Part model, mm, in its own coordinate system. A direction names the side the tool comes from. Round coordinates to 2 decimals unless told otherwise and drop trailing zeros. Loops run counter-clockwise (first coordinate to the right, second up) from the corner with the lowest first, then second, coordinate; pieces in that order, holes last.
from build123d import *

# Parameters (mm, degrees)
SKETCH_1_R               = 30
SKETCH_1_R_2             = 2.5
EXTRUDE_1_DEPTH          = 17
SKETCH_2_R               = 16
CUT_EXTRUDE_1_DEPTH      = 18
PATTERN_CIRCULAR_1_COUNT = 3
SKETCH_4_R               = 11
EXTRUDE_3_DEPTH          = 14
SKETCH_5_R               = 5
CUT_EXTRUDE_2_DEPTH      = 32
SKETCH_6_W               = 4
SKETCH_6_H               = 2.5
CUT_EXTRUDE_3_DEPTH      = 32
SKETCH_7_R               = 13
EXTRUDE_4_DEPTH          = 4
EXTRUDE_5_DEPTH          = 35
SKETCH_10_R              = 13
SKETCH_10_R_2            = 11
EXTRUDE_8_DEPTH          = 3
FILLET_1_R               = 5


with BuildPart() as part:
    # 草图1 → 凸台-拉伸1 (new body)
    with BuildSketch(Plane.XY):
        Circle(SKETCH_1_R)
        with Locations((-5.952838037, 22.216294005)):
            Circle(SKETCH_1_R_2, mode=Mode.SUBTRACT)
        with Locations((5.952838037, 22.216294005)):
            Circle(SKETCH_1_R_2, mode=Mode.SUBTRACT)
        with Locations((22.216294005, -5.952838037)):
            Circle(SKETCH_1_R_2, mode=Mode.SUBTRACT)
        with Locations((16.263455967, -16.263455967)):
            Circle(SKETCH_1_R_2, mode=Mode.SUBTRACT)
        with Locations((-16.263455967, -16.263455967)):
            Circle(SKETCH_1_R_2, mode=Mode.SUBTRACT)
        with Locations((-22.216294005, -5.952838037)):
            Circle(SKETCH_1_R_2, mode=Mode.SUBTRACT)
    extrude(amount=EXTRUDE_1_DEPTH)

    # 草图2 → 切除-拉伸1 (cut, through all)
    with BuildSketch(Plane.XY.offset(17)):
        with Locations((25.980762114, 15)):
            Circle(SKETCH_2_R)
    cut_extrude_1 = extrude(amount=-CUT_EXTRUDE_1_DEPTH, mode=Mode.SUBTRACT)

    # 阵列(圆周)1: 切除-拉伸1 ×3 about axis
    pattern_circular_1_axis = Axis((0, 0, 0), (0, 0, 1))
    for i in range(1, PATTERN_CIRCULAR_1_COUNT):
        add(cut_extrude_1.rotate(pattern_circular_1_axis, i * 360 / PATTERN_CIRCULAR_1_COUNT), mode=Mode.SUBTRACT)

    # 草图4 → 凸台-拉伸3 (add)
    with BuildSketch(Plane.XY.offset(17)):
        Circle(SKETCH_4_R)
    extrude(amount=EXTRUDE_3_DEPTH)

    # 草图5 → 切除-拉伸2 (cut, through all)
    with BuildSketch(Plane.XY.offset(31)):
        Circle(SKETCH_5_R)
    extrude(amount=-CUT_EXTRUDE_2_DEPTH, mode=Mode.SUBTRACT)

    # 草图6 → 切除-拉伸3 (cut, through all)
    with BuildSketch(Plane.XY.offset(31)):
        with Locations((0, 5)):
            Rectangle(SKETCH_6_W, SKETCH_6_H)
    extrude(amount=-CUT_EXTRUDE_3_DEPTH, mode=Mode.SUBTRACT)

    # 草图7 → 凸台-拉伸4 (add)
    with BuildSketch(Plane(origin=(0, 0, 0), x_dir=(-1, 0, 0), z_dir=(0, 0, -1))):
        Circle(SKETCH_7_R)
        with BuildLine():
            Line((-2, 4.582575695), (-2, 6.25))
            Line((-2, 6.25), (2, 6.25))
            Line((2, 6.25), (2, 4.582575695))
            ThreePointArc((2, 4.582575695), (0, -5), (-2, 4.582575695))
        make_face(mode=Mode.SUBTRACT)
    extrude(amount=EXTRUDE_4_DEPTH)

    # 草图8 → 凸台-拉伸5 (add)
    with BuildSketch(Plane(origin=(0, 0, -4), x_dir=(-1, 0, 0), z_dir=(0, 0, -1))):
        with BuildLine():
            Line((-2, 4.582575695), (-2, 6.25))
            Line((-2, 6.25), (2, 6.25))
            Line((2, 6.25), (2, 4.582575695))
            ThreePointArc((2, 4.582575695), (0, 5), (-2, 4.582575695))
        make_face()
    extrude(amount=-EXTRUDE_5_DEPTH)

    # 草图10 → 凸台-拉伸8 (add)
    with BuildSketch(Plane.XY.offset(17)):
        Circle(SKETCH_10_R)
        Circle(SKETCH_10_R_2, mode=Mode.SUBTRACT)
    extrude(amount=EXTRUDE_8_DEPTH)

    # 圆角1
    fillet_1_edges = [part.edges().sort_by_distance(p)[0] for p in [
        (14.575409833, 26.221316294, 8.5),
        (29.996030948, -0.487982961, 8.5),
        (-29.996030948, -0.487982961, 8.5),
        (-14.575409833, 26.221316294, 8.5),
        (15.420621114, -25.733333333, 8.5),
        (-15.420621114, -25.733333333, 8.5),
    ]]
    fillet(fillet_1_edges, radius=FILLET_1_R)


solid = part.part
1) Tool access for faces 1 (the face through (18.573, -17.221, 8.381)), 2 (the face through (-10.316, -7.91, 18.479)), 3 (the face through (-7, -14, 0)): list every direction of +Z, -Z, +X, -X, +Y, -Y with a clear straight run to the whole face (end or side of a thin tool).
Values:
face 1: +Z, -Z
face 2: +Z
face 3: -Z
2) Slice it at A-A, the plane x = 0. Give the cut face in (y, z), then the cut area to 3 significant figures.
Values:
outline: (-14, 0) - (-13, 0) - (-13, -4) - (-5, -4) - (-5, 31) - (-11, 31) - (-11, 20) - (-13, 20) - (-13, 17) - (-14, 17) - close; (5, -4) - (13, -4) - (13, 0) - (30, 0) - (30, 17) - (13, 17) - (13, 20) - (11, 20) - (11, 31) - (5, 31) - close
area: 822 mm2
3) Slice it at D-D, the plane y = -18. Give the cut face in (x, z) (3 decimals).
Values:
outline: (-24, 0) - (-18.062, 0) - (-18.062, 17) - (-24, 17) - close; (-14.465, 0) - (-10.583, 0) - (-10.583, 17) - (-14.465, 17) - close; (10.583, 0) - (14.465, 0) - (14.465, 17) - (10.583, 17) - close; (18.062, 0) - (24, 0) - (24, 17) - (18.062, 17) - close
4) Drop flat-ended pins along their axis: pin 1 Ø5 at (x, y) = (-6.5, 18.5) entering from -Z; pin 2 Ø12 at (y, z) = (0.5, 0) entering from -X; pin 3 Ø4.5 at (x, y) = (-5.95, 22.22) entering from -Z; pin 4 Ø6.5 at (x, y) = (-22.22, -5.95) entering from +Z. Give the stop position or say it passes through.
Values:
pin 1: stops at z = 0
pin 2: stops at x = -29.27
pin 3: passes through
pin 4: stops at z = 17
5) Mould opens along X. For faces 4 (the face through (0, -14, 9)), 5 (the face through (10.316, -7.91, -1.972)), 6 (the face through (-7, -14, 17)) say: released by +X, released by -X, zero draft, split by the parting line, or undercut.
Values:
face 4: undercut
face 5: split by the parting line
face 6: zero draft
6) Wall check: line 1 along X through (y, z) = (-6, 3); line 2 along X through (y, z) = (4, 5); line 3 along X through (y, z) = (2, 6.5). Give the ranges that are in metal, low to high.
Values:
line 1: x = -29.29 to -24.72, -19.72 to 19.72, 24.72 to 29.29
line 2: x = -14.36 to -3, 3 to 14.36
line 3: x = -16.65 to -4.58, 4.58 to 16.65
7) Slice it at B-B, the plane y = 0. Give the cut face in (x, z), then the cut area to 3 significant figures.
Values:
outline: (-20.41, 0) - (-13, 0) - (-13, -4) - (-5, -4) - (-5, 31) - (-11, 31) - (-11, 20) - (-13, 20) - (-13, 17) - (-20.41, 17) - close; (5, -4) - (13, -4) - (13, 0) - (20.41, 0) - (20.41, 17) - (13, 17) - (13, 20) - (11, 20) - (11, 31) - (5, 31) - close
area: 768 mm2
8) Slice it at C-C, the plane z = 27.5. Give the cut face in (x, y), then the cut area to 3 significant figures.
Values:
outline: circle Ø22 at (0, 0); hole circle Ø10 at (0, 0)
area: 302 mm2
